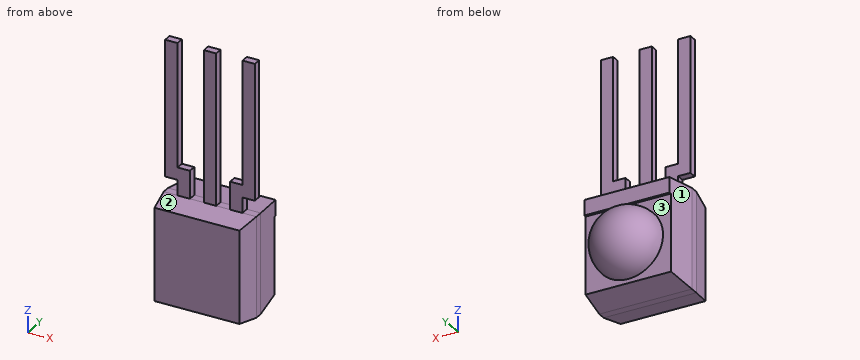
from build123d import *

# Parameters (mm, degrees)
SKETCH1_W           = 6
SKETCH1_H           = 6.5
BOSS_EXTRUDE1_DEPTH = 4
SKETCH2_W           = 0.8
SKETCH2_H           = 0.5
BOSS_EXTRUDE2_DEPTH = 1
SKETCH3_W           = 0.8
SKETCH3_H           = 8.8
BOSS_EXTRUDE3_DEPTH = 0.5
REVOLVE1_ANGLE      = 180
SKETCH5_W           = 6
SKETCH5_H           = 1.25
BOSS_EXTRUDE4_DEPTH = 0.15
CUT_EXTRUDE1_DEPTH  = 13.004270074
CUT_EXTRUDE2_DEPTH  = 16.664131


with BuildPart() as part:
    # Sketch1 → Boss-Extrude1 (new body)
    with BuildSketch(Plane(origin=(0, 0, 0), x_dir=(1, 0, 0), z_dir=(0, 1, 0))):
        Rectangle(SKETCH1_W, SKETCH1_H)
    extrude(amount=BOSS_EXTRUDE1_DEPTH)

    # Sketch2 → Boss-Extrude2 (add)
    with BuildSketch(Plane.XY.offset(3.25)):
        with Locations((-1.7, 1.75)):
            Rectangle(SKETCH2_W, SKETCH2_H)
        with Locations((0, 1.75)):
            Rectangle(SKETCH2_W, SKETCH2_H)
        with Locations((1.7, 1.75)):
            Rectangle(SKETCH2_W, SKETCH2_H)
    extrude(amount=BOSS_EXTRUDE2_DEPTH)

    # Sketch3 → Boss-Extrude3 (add)
    with BuildSketch(Plane(origin=(0, 2, 0), x_dir=(1, 0, 0), z_dir=(0, 1, 0))):
        Polygon((-1.3, -4.25), (-1.3, -5.05), (-2.1, -5.05), (-2.1, -13.05), (-2.9, -13.05), (-2.9, -4.25), (-2.1, -4.25), align=None)
        with Locations((0, -8.65)):
            Rectangle(SKETCH3_W, SKETCH3_H)
        Polygon((1.3, -4.25), (2.9, -4.25), (2.9, -13.05), (2.1, -13.05), (2.1, -5.05), (1.3, -5.05), align=None)
    extrude(amount=-BOSS_EXTRUDE3_DEPTH)

    # Sketch4 → Revolve1 (revolve)
    with BuildSketch(Plane(origin=(0, 4, 0), x_dir=(1, 0, 0), z_dir=(0, 1, 0))):
        with BuildLine():
            Line((0, 2.75), (0, -1.75))
            ThreePointArc((0, -1.75), (-2.25, 0.5), (0, 2.75))
        make_face()
    revolve(axis=Axis((0, 4, -2.75), (0, 0, -1)), revolution_arc=REVOLVE1_ANGLE)

    # Sketch5 → Boss-Extrude4 (add)
    with BuildSketch(Plane(origin=(0, 4, 0), x_dir=(1, 0, 0), z_dir=(0, 1, 0))):
        with Locations((0, -2.625)):
            Rectangle(SKETCH5_W, SKETCH5_H)
    extrude(amount=BOSS_EXTRUDE4_DEPTH)

    # Sketch6 → Cut-Extrude1 (cut, through all)
    with BuildSketch(Plane.XY.offset(3.25)):
        Polygon((-3, 2), (-2.75, 4.15), (-3, 4.15), align=None)
        Polygon((-3, 1.5), (-2.75, 0), (-3, 0), align=None)
        Polygon((3, 0), (3, 1.5), (2.75, 0), align=None)
        Polygon((3, 4.15), (3, 2), (2.75, 4.15), align=None)
    extrude(amount=-CUT_EXTRUDE1_DEPTH, mode=Mode.SUBTRACT)

    # Sketch7 → Cut-Extrude2 (cut, through all)
    with BuildSketch(Plane.ZY.offset(3)):
        Polygon((3.25, 2), (3.25, 4.15), (3, 4.15), align=None)
        Polygon((3.25, 1.5), (3.25, 0), (3, 0), align=None)
        Polygon((-3, 0), (-3.25, 1.5), (-3.25, 0), align=None)
        Polygon((-3, 4.15), (-3.25, 2), (-3.25, 4.15), align=None)
    extrude(amount=-CUT_EXTRUDE2_DEPTH, mode=Mode.SUBTRACT)


solid = part.part
Source: CAD feature listing. Evaluate the final solid. Frame: model axes, mm. Face numbers are marked on the shaded views. Coordinates: 2 decimals unless noted, no trailing zeros. Write each loop counter-clockwise with the first axis right and the second up, starting at its lowest first coordinate (ties: lowest second). Pieces come first, ordered by that corner, then holes. Notation, with made-up numbers: M -35.5,26.25 L -24.5,26.25 A19 cw -24.5,38.25 Z; hole C 42.5,75 d2. An arc over 180 degrees is marked long. Use a Markdown table: item, result.
1) Ray query, L1, parallel to Y at x = 2.5, z = 8.5; L2, parallel to Y at x = 2.25, z = -2.5; L3, parallel to Z at x = -0.75, y = 3.5. Return the intervals inside material, ascending.
Conclusion:
| item | result |
|---|---|
| L1 | y = 1.5 to 2 |
| L2 | y = 0 to 4 |
| L3 | z = -3.08 to 3.08 |
2) Section A-A, the plane z = 6. Output: boundary loops of the cut face in (x, y), then the cut area to 3 significant figures.
Conclusion:
| item | result |
|---|---|
| outline | M -2.9,1.5 L -2.1,1.5 L -2.1,2 L -2.9,2 Z; M -0.4,1.5 L 0.4,1.5 L 0.4,2 L -0.4,2 Z; M 2.1,1.5 L 2.9,1.5 L 2.9,2 L 2.1,2 Z |
| area | 1.20 mm^2 |
3) Mould query, pull axis Z, two halves, no side actions, for the marked faces 1, 2 and 3. Classes: pulls with the +Z half, pulls with the -Z half, needs draft (parallel to the pull), parting line crosses it, or undercut.
Conclusion:
| item | result |
|---|---|
| face 1 | needs draft |
| face 2 | pulls with the +Z half |
| face 3 | undercut |
4) First-contact query: pin 1 Ø0.8 at (x, z) = (2, 8.5) entering from +Y; pin 2 Ø2 at (x, z) = (-2, 2.5) entering from +Y; pin 3 Ø1.5 at (x, y) = (2.5, 3) entering from +Z. Flat tips, straight axial feed; report the tip coordinate or a pass-through.
Conclusion:
| item | result |
|---|---|
| pin 1 | stops at y = 2 |
| pin 2 | stops at y = 4.15 |
| pin 3 | stops at z = 3.22 |
5) Section C-C, the plane y = 1.75. Output: boundary loops of the cut face in (x, z).
Conclusion:
| item | result |
|---|---|
| outline | M -3,-3.25 L 3,-3.25 L 3,3.25 L 2.1,3.25 L 2.1,4.25 L 2.9,4.25 L 2.9,13.05 L 2.1,13.05 L 2.1,5.05 L 1.3,5.05 L 1.3,3.25 L 0.4,3.25 L 0.4,13.05 L -0.4,13.05 L -0.4,3.25 L -1.3,3.25 L -1.3,5.05 L -2.1,5.05 L -2.1,13.05 L -2.9,13.05 L -2.9,4.25 L -2.1,4.25 L -2.1,3.25 L -3,3.25 Z |
6) Section D-D, the plane z = -0.75. Output: boundary loops of the cut face in (x, y).
Conclusion:
| item | result |
|---|---|
| outline | M -3,1.5 L -2.75,0 L 2.75,0 L 3,1.5 L 3,2 L 2.77,4 L 2.24,4 A2.24 ccw -2.24,4 L -2.77,4 L -3,2 Z |
7) Section B-B, the plane x = -2.5. Output: boundary loops of the cut face in (y, z), then the cut area to 3 significant figures.
Conclusion:
| item | result |
|---|---|
| outline | M 0,-3 L 1.5,-3.25 L 2,-3.25 L 4,-3.02 L 4,2 L 4.15,2 L 4.15,3 L 2,3.25 L 1.5,3.25 L 0,3 Z; M 1.5,4.25 L 2,4.25 L 2,13.05 L 1.5,13.05 Z |
| area | 29.7 mm^2 |
